from build123d import *

# Parameters (mm, degrees)
F1_DEPTH = 25.4


with BuildPart() as f1:
    # F0 (on Front) → F1 (new body)
    with BuildSketch(Plane.XZ):
        Polygon((-36.657058, 13.813218), (-38.634382, 10.649496), (-29.441338, 10.649496), (-16.448003, 2.52867), (-21.472151, -5.509975), (-23.449069, -13.3819), (-26.721189, -20.258428), (-26.721189, -24.452301), (-26.721189, -37.052132), (-25.958963, -40.006805), (-19.755764, -40.006805), (-18.349815, -37.052132), (-19.755764, -33.562165), (-19.755764, -28.500162), (-19.755764, -21.963648), (-13.268332, -17.527793), (-7.529761, -20.258428), (-7.529761, -37.052132), (-7.529761, -40.006805), (-6.040169, -43.91915), (0, -43.91915), (2.030398, -42.189743), (0, -37.052132), (-0.887454, -32.503918), (-0.887454, -30.455308), (-0.887454, -28.034225), (0, -20.398496), (3.290899, -20.780977), (5.537732, -20.780977), (7.213868, -20.780977), (8.238172, -20.780977), (9.169359, -19.932901), (10.193664, -19.932901), (10.752375, -18.536123), (11.795948, -18.953552), (11.795948, -25.892494), (13.452818, -27.847987), (13.452818, -37.052132), (15.222071, -40.006805), (16.70198, -40.931748), (21.69138, -40.931748), (24.033716, -40.006805), (22.866973, -37.052132), (20.397942, -35.508989), (20.397942, -32.503918), (20.397942, -26.903253), (20.9637, -22.035432), (20.9637, -17.422371), (20.397942, -14.633874), (20.844123, -10.794904), (21.209698, -7.64946), (21.209698, -5.152992), (19.460583, -2.141417), (19.460583, 0), (18.456725, 3.212494), (18.777084, 5.968888), (20.397942, 8.562263), (20.397942, 10.016422), (20.677842, 12.4247), (22.866973, 11.056494), (23.722101, 12.4247), (26.054654, 16.156789), (26.054654, 17.378049), (26.475677, 21.000561), (26.677313, 22.735452), (19.279403, 27.35914), (16.70198, 25.764998), (14.486361, 27.149758), (12.621277, 27.366526), (10.876146, 27.569352), (9.169359, 27.767721), (7.452843, 27.967221), (5.537732, 27.767721), (3.290899, 27.151791), (-6.040169, 23.721304), (-6.040169, 21.000561), (-5.347158, 17.378049), (-5.347158, 13.867774), (-4.617267, 10.016422), (-0.887454, 14.524676), (-0.887454, 7.371743), (-1.922802, 8.018835), (-3.070138, 8.152183), (-4.341321, 8.299925), (-6.040169, 8.018835), (-7.529761, 6.933809), (-9.373561, 5.921237), (-25.958963, 13.813218), align=None)
        Polygon((-0.887454, -32.503918), (0, -37.052132), (0.515232, -34.941698), (2.030398, -35.117797), (3.290899, -35.264297), (4.526607, -35.407916), (4.526607, -34.476705), (4.526607, -33.562165), (4.025185, -31.611435), (3.290899, -30.455308), (2.030398, -29.247591), (1.231548, -28.034225), (0.515232, -26.903253), (0.515232, -24.878059), (0.515232, -23.517057), (0.515232, -21.583002), (0, -20.398496), (-0.887454, -28.034225), (-0.887454, -30.455308), align=None)
    extrude(amount=F1_DEPTH)


solid = f1.part
Read the model definition and answer for the solid it produces. Units are mm, in the model's axes. A direction names the side the tool comes from. Coordinates: 2 decimals unless noted, no trailing zeros. Write each loop counter-clockwise with the first axis right and the second up, starting at its lowest first coordinate (ties: lowest second). Pieces come first, ordered by that corner, then holes. Notation, with made-up numbers: (-1, 87.25) -> (45, 87.25) arc R24 ccw to (45, 106.25) -> close; hole circle Ø8 at (-32.5, 26.5). An arc over 180 degrees is marked (long way). Return JSON: item names as keys, results as strings.
(1) The part is cut by section B-B on z = -15.5. Give the vertices of the cut face in (x, y), then the cut area to 3 significant figures.
Answers below:
{"outline": "(-24.46, -25.4) -> (20.57, -25.4) -> (20.57, 0) -> (-24.46, 0) -> close", "area": "1,140 mm^2"}
(2) Which of the six approach directions +Z, -Z, +X, -X, +Y, -Y give full straight-line access (tool end or side, diameter ignored) to faces 5 (the flat face through (11.796, -13, -22)), 6 (the flat face through (0.254, -12.522, -36.012)), 7 (the flat face through (23.46, -12.52, -38.55))?
Answers below:
{"face 5": "-Z, +Y, -Y", "face 6": "+Y, -Y", "face 7": "+X, +Y, -Y"}
(3) For a pull along X with two mould halves and no side action, classify faces 1 (the flat face through (-26.345, -12.522, -38.509)), 2 (the flat face through (-31, -13, 13.813)), 3 (the flat face through (0.515, -13, -24)), 4 (the flat face through (19.58, -12.52, 7.25)) as pulls with the +X half, pulls with the -X half, needs draft (parallel to the pull), parting line crosses it, or undercut.
Answers below:
{"face 1": "pulls with the -X half", "face 2": "needs draft", "face 3": "undercut", "face 4": "pulls with the +X half"}
(4) Each of these flat-tipped pins is pushed along its axis until it touches: P1, Ø10, axis at y = -14.5, z = -17.5, coming from the -X side; P2, Ø4, axis at x = 18.5, y = -13, coming from the -Z side; P3, Ø5, axis at x = -12.5, z = -28, coming from the -Y side; P4, Ø5, axis at x = -21.5, y = -18, coming from the -Z side. Where does it stop, or does it pass through?
Answers below:
{"P1": "x = -26.72", "P2": "z = -40.93", "P3": "through", "P4": "z = -40.01"}
(5) Consider line 1 along X through (y, z) = (-16.5, -31); line 2 along X through (y, z) = (-2.25, -19.5); line 3 along Z through (x, y) = (12.5, -21.5). Determine where each line is inside the solid, lowest interval first. Write a range as from..to.
Answers below:
{"line 1": "-26.72..-19.76, -7.53..3.64, 13.45..20.4", "line 2": "-26.36..-16.15, -9.12..10.37, 11.8..20.96", "line 3": "-26.72..27.38"}
(6) The part is cut by section A-A on x = -31. Give the vertices of the cut face in (y, z).
Answers below:
{"outline": "(-25.4, 10.65) -> (0, 10.65) -> (0, 13.81) -> (-25.4, 13.81) -> close"}
